Autodesk Inventor part; units mm, degrees
ref_plane "Work Plane1" through (0, 0, 16) normal (0, 0, 1) x (1, 0, 0)
ref_plane "YZ Plane" through (0, 0, 0) normal (1, 0, 0) x (0, 1, 0)
ref_plane "XZ Plane" through (0, 0, 0) normal (0, 1, 0) x (-1, 0, 0)
sketch "Sketch1" plane through (0, 0, 0) normal (0, 0, 1) x (1, 0, 0)
  circle A0 centre (0, 0) radius 47.5
  circle A1 centre (0, 0) radius 4.25
  circle A2 centre (25, 0) radius 2.5
  circle A3 centre (12.5, 21.6506) radius 2.5
  circle A4 centre (-12.5, 21.6506) radius 2.5
  circle A5 centre (-25, 0) radius 2.5
  circle A6 centre (-12.5, -21.6506) radius 2.5
  circle A7 centre (12.5, -21.6506) radius 2.5
  dimension "d0" = 95
  dimension "d1" = 8.5
  dimension "d2" = 5
  dimension "d3" = 25
  dimension "d6" = 360
extrude "Extrusion1" add sketch "Sketch1" along normal blind 54
ref_plane "Work Plane1" through (0, 0, 16) normal (0, 0, 1) x (1, 0, 0)
sketch "Sketch2" plane through (0, 0, 16) normal (0, 0, 1) x (1, 0, 0)
  circle A0 centre (0, 0) radius 47.5
  line L0 (44.1588, 17.5) -> (51.1588, 17.5)
  line L1 (51.1588, 17.5) -> (51.1588, -17.5)
  line L2 (51.1588, -17.5) -> (44.1588, -17.5)
  line L3 (44.1588, -17.5) -> (44.1588, 17.5)
  point P0 (44.1588, 0)
  dimension "d11" = 7
  dimension "d12" = 35
extrude "Extrusion2" add sketch "Sketch2" along normal mid plane 25 contours A0 L0 L1 L2
sketch "Sketch3" plane through (51.1588, -17.5, 28.5) normal (1, 0, 0) x (0, 0, -1)
  line L0 (-17.5, 47.5) -> (42.5, 47.5)
  line L1 (42.5, 47.5) -> (42.5, -12.5)
  line L2 (42.5, -12.5) -> (-17.5, -12.5)
  line L3 (-17.5, -12.5) -> (-17.5, 47.5)
  line L4 (25, 35) -> (0, 35)
  line L5 (0, 0) -> (0, 35)
  line L6 (25, 0) -> (0, 0)
  line L7 (25, 35) -> (25, 0)
  line L8 (25, 35) -> (25, 0)
  point P0 (28.5, 17.5)
  point P1 (-17.5, 17.5)
  point P2 (25, 17.5)
  point P3 (12.5, 47.5)
  point P4 (12.5, 35)
  dimension "d15" = 60
  dimension "d16" = 60
extrude "Extrusion3" add sketch "Sketch3" along normal blind 10 contours L0 L1 L2 L3 | L7 L6 L5 L4
fillet "Fillet1" radius 20 4 edges at (56.1588, 30, 46) (56.1588, 30, -14) (56.1588, -30, -14) (56.1588, -30, 46)
sketch "Sketch4" plane through (61.1588, -17.5, 28.5) normal (1, 0, 0) x (0, 0, -1)
  line L0 (2.5, 32.5) -> (22.5, 32.5) construction
  line L1 (22.5, 32.5) -> (22.5, 2.5) construction
  line L2 (22.5, 2.5) -> (2.5, 2.5) construction
  line L3 (2.5, 2.5) -> (2.5, 32.5) construction
  line L4 (22.5, 47.5) -> (2.5, 47.5)
  line L5 (42.5, 7.5) -> (42.5, 27.5)
  circle A0 centre (2.5, 32.5) radius 2.5
  circle A1 centre (22.5, 32.5) radius 2.5
  circle A2 centre (2.5, 2.5) radius 2.5
  circle A3 centre (22.5, 2.5) radius 2.5
  point P0 (28.5, 17.5)
  point P1 (22.5, 17.5)
  point P2 (42.5, 17.5)
  point P3 (12.5, 32.5)
  point P4 (12.5, 47.5)
  dimension "d20" = 20
  dimension "d21" = 30
  dimension "d22" = 5
  dimension "d23" = 5
  dimension "d24" = 5
  dimension "d25" = 5
extrude "Extrusion4" cut sketch "Sketch4" against normal blind 30
sketch "Sketch5" plane through (61.1588, -17.5, 28.5) normal (1, 0, 0) x (0, 0, -1)
  circle A0 centre (12.5, 17.5) radius 14
  line L0 (42.5, 7.5) -> (42.5, 27.5)
  line L1 (2.5, -12.5) -> (22.5, -12.5)
  point P0 (28.5, 17.5)
  point P1 (12.5, -12.5)
  point P2 (42.5, 17.5)
  dimension "d28" = 28
extrude "Extrusion5" cut sketch "Sketch5" against normal blind 13
sketch "Sketch6" plane through (0, 0, 54) normal (0, 0, 1) x (1, 0, 0)
  circle A0 centre (0, 0) radius 47.5
extrude "Extrusion6" cut sketch "Sketch6" against normal blind 10
sketch "Sketch7" plane through (0, 0, 44) normal (0, 0, 1) x (1, 0, 0)
  circle A0 centre (0, 0) radius 47.5
  circle A1 centre (0, 0) radius 42.5
  circle A2 centre (0, 0) radius 17.5
  dimension "d33" = 5
  dimension "d34" = 35
extrude "Extrusion7" cut sketch "Sketch7" against normal blind 15 contours A1
sketch "Sketch8" plane through (0, 0, 44) normal (0, 0, 1) x (1, 0, 0)
  circle A0 centre (0, 0) radius 13.5
  dimension "d37" = 27
extrude "Extrusion8" cut sketch "Sketch8" against normal blind 10
sketch "Sketch9" plane through (0, 0, 34) normal (0, 0, 1) x (1, 0, 0)
  circle A0 centre (0, 9.525) radius 1.5
  circle A1 centre (-8.2489, 4.7625) radius 1.5
  circle A2 centre (-8.2489, -4.7625) radius 1.5
  circle A3 centre (0, -9.525) radius 1.5
  circle A4 centre (8.2489, -4.7625) radius 1.5
  circle A5 centre (8.2489, 4.7625) radius 1.5
  point P0 (0, 0)
  dimension "d40" = 3
  dimension "d41" = 9.525
  dimension "d44" = 360
extrude "Extrusion9" cut sketch "Sketch9" against normal blind 15
sketch "Sketch10" plane through (0, 0, 0) normal (1, 0, 0) x (0, 1, 0)
  line L0 (-13.5, 34) -> (13.5, 34)
  line L1 (-13.5, 44) -> (13.5, 44)
  circle A0 centre (0, 36.75) radius 1.5
  circle A1 centre (0, 41.85) radius 1.5
  line L2 (0, 38.25) -> (0, 40.35)
  line L3 (-13.5, 34) -> (13.5, 34)
  line L4 (0, 34) -> (0, 35.25)
  point P0 (0, 0)
  dimension "d49" = 3
  dimension "d48" = 3
  dimension "d50" = 2.1
  dimension "d52" = 1.25
extrude "Extrusion10" cut sketch "Sketch10" against normal through all
sketch "Sketch11" plane through (51.1588, -17.5, 28.5) normal (-1, 0, 0) x (0, 0, 1)
  line L0 (-80.8261, -70.2881) -> (37.6957, -70.2881)
  line L1 (37.6957, -70.2881) -> (37.6957, 87.9511)
  line L2 (37.6957, 87.9511) -> (-80.8261, 87.9511)
  line L3 (-80.8261, 87.9511) -> (-80.8261, -70.2881)
  point P0 (-28.5, 17.5)
extrude "Extrusion11" cut sketch "Sketch11" along normal through all
equation "\"d26\" = d21"
properties part number "AA036" material "ABS Plastic"
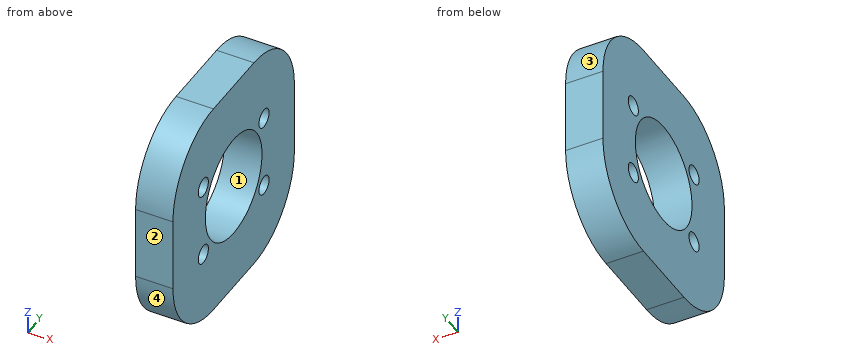
Check sheet for the modelled part. Datum: model origin and axes. Units: mm. Face numbers are marked on the shaded views. Give positions to 0.01 mm unless a question says otherwise; leave off trailing zeros. Write each loop counter-clockwise with the first axis right and the second up, starting at its lowest first coordinate (ties: lowest second). Pieces come first, ordered by that corner, then holes. Notation, with made-up numbers: (6.5, 28.5) -> (28.5, 28.5) arc R12 cw to (28.5, 35.5) -> close; hole circle Ø2 at (-11, 44). An arc over 180 degrees is marked (long way). Use one line per item in the form item = value. Start each with the question number.
1. Mould release check, pull along Z, two halves, no side actions. Record for the marked faces 1, 2, 3 and 4: pulls with the +Z half, pulls with the -Z half, needs draft (parallel to the pull), parting line crosses it, or undercut.
2. Thickness scan on line 1 along Y through (x, z) = (56.5, 6); line 2 along Y through (x, z) = (59.75, 16.5); line 3 along Y through (x, z) = (53, 7). Record the ranges inside material, lowest first. Write a range as from..to.
3. Go/stop test with flat-tipped pins: P1, Ø6, axis at y = 15, z = 26, coming from the -X side; P2, Ø3, axis at x = 54.5, z = -7, coming from the +Y side. Record where each tip stops, or that it passes through.
4. Section check A-A (y = 0). Record the cut outline in (x, z), and give its area (3 significant figures).
5. Section check C-C (x = 59.25). Record the cut outline in (y, z).
6. Section check D-D (y = -15). Record the cut outline in (x, z), and give its area (3 significant figures).
7. Section check B-B (z = 16). Record the cut outline in (x, y).
Conclusion:
q1.face_1 = undercut
q1.face_2 = needs draft
q1.face_3 = pulls with the +Z half
q1.face_4 = pulls with the -Z half
q2.line_1 = -30..-17.5, -12.5..-9.8, 9.8..12.5, 17.5..30
q2.line_2 = -30..-13.99, 13.99..30
q2.line_3 = -30..-17.29, -12.71..-10.72, 10.72..12.71, 17.29..30
q3.P1 = 51.16
q3.P2 = 26.36
q4.outline = (51.16, -14) -> (61.16, -14) -> (61.16, 2) -> (51.16, 2) -> close; (51.16, 30) -> (61.16, 30) -> (61.16, 46) -> (51.16, 46) -> close
q4.area = 320 mm²
q5.outline = (-30, 6) arc R20 ccw to (-10, -14) -> (10, -14) arc R20 ccw to (30, 6) -> (30, 26) arc R20 ccw to (10, 46) -> (-10, 46) arc R20 ccw to (-30, 26) -> close; hole circle Ø5 at (-15, 6); hole circle Ø5 at (-15, 26); hole circle Ø28 at (0, 16); hole circle Ø5 at (15, 6); hole circle Ø5 at (15, 26)
q6.outline = (51.16, -13.36) -> (61.16, -13.36) -> (61.16, 3.5) -> (51.16, 3.5) -> close; (51.16, 8.5) -> (61.16, 8.5) -> (61.16, 23.5) -> (51.16, 23.5) -> close; (51.16, 28.5) -> (61.16, 28.5) -> (61.16, 45.36) -> (51.16, 45.36) -> close
q6.area = 487 mm²
q7.outline = (51.16, -30) -> (61.16, -30) -> (61.16, -14) -> (51.16, -14) -> close; (51.16, 14) -> (61.16, 14) -> (61.16, 30) -> (51.16, 30) -> close
